For this review, take the finished solid that the model builds, in its own axes (mm). Face numbers are marked on the shaded views. A direction names the side the tool comes from. Give positions to 0.01 mm unless a question says otherwise; leave off trailing zeros. Order: outer loops, then holes, each group sorted by start corner. A loop starts at its lowest first (then second) coordinate and runs counter-clockwise, first axis right, second up.
Item 1: Consider section A-A (x = 0). Give the boundary of the cut face in (y, z).
Item 2: Machinability: for the marked faces 4, 5 and 6, which of the approach directions +Z, -Z, +X, -X, +Y, -Y give a long, thin tool a straight path to every point of the face, cutting with its end or side? Answer none if there is none.
Item 3: For P1, Ø2, axis at y = -0.5, z = -20.5, coming from the +X side; P2, Ø1, axis at x = 5, y = 1, coming from the +Z side; P3, Ø6, axis at y = -0.5, z = -13, coming from the +X side, all flat-tipped, find the tip position at first contact; note any pin that passes through.
Item 4: The part is to be moulded in two halves that separate along Z. For the marked faces 1, 2 and 3, say which applies: released by +Z, released by -Z, zero draft, split by the parting line, or undercut.
Item 5: Consider section B-B (z = -31). Give the boundary of the cut face in (x, y).
Item 6: Consider section D-D (x = -7). Give the boundary of the cut face in (y, z).
Item 7: For probe 1 along Z at (x, y) = (0, 0.25); probe 2 along X at (y, z) = (-4.5, -9.5); probe 3 along Z at (x, y) = (-4, -2.5), list the stretches that pass through material, from the lowest coordinate up.
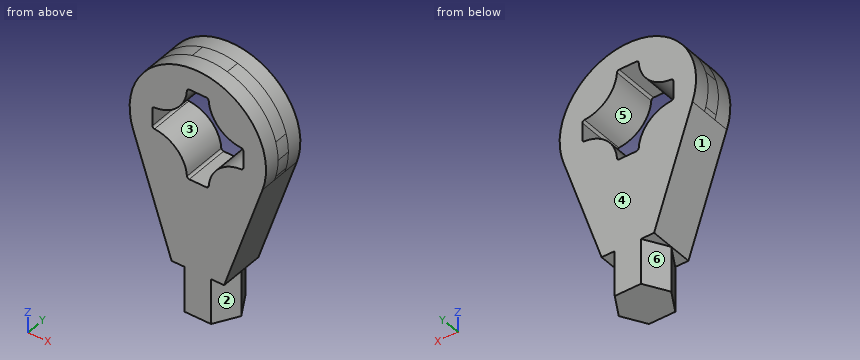
```python
from build123d import *

# Parameters (mm, degrees)
F1_DEPTH   = 3
F5_DEPTH   = 10
F7_DEPTH   = 3
F1_FACE1_R = 15
F8_DEPTH   = 3.5
F1_FACE_R  = 15
F9_DEPTH   = 3.5
F11_R      = 0.5


with BuildPart() as f1:
    # F0 (on Front) → F1 (new body)
    with BuildSketch(Plane.XZ):
        with BuildLine():
            Line((-10, -2.375), (-10, 2.375))
            ThreePointArc((-10, 2.375), (-12.3664158462, 2.7515035323), (-14.4991362367, 3.8438325133))
            ThreePointArc((-14.4991362367, 3.8438325133), (-15, 0), (-14.4991362367, -3.8438325133))
            ThreePointArc((-14.4991362367, -3.8438325133), (-12.3664158462, -2.7515035323), (-10, -2.375))
        make_face()
        with BuildLine():
            Line((-10, 10), (-2.375, 10))
            ThreePointArc((-2.375, 10), (-2.7515035323, 12.3664158462), (-3.8438325133, 14.4991362367))
            ThreePointArc((-3.8438325133, 14.4991362367), (-10.6066017178, 10.6066017178), (-14.4991362367, 3.8438325133))
            ThreePointArc((-14.4991362367, 3.8438325133), (-12.3664158462, 2.7515035323), (-10, 2.375))
            Line((-10, 2.375), (-10, 10))
        make_face()
        with BuildLine():
            ThreePointArc((-10, 2.375), (-4.6083107935, 4.6083107935), (-2.375, 10))
            Line((-2.375, 10), (-10, 10))
            Line((-10, 10), (-10, 2.375))
        make_face()
        with BuildLine():
            Line((-2.375, 10), (2.375, 10))
            ThreePointArc((2.375, 10), (2.7515035323, 12.3664158462), (3.8438325133, 14.4991362367))
            ThreePointArc((3.8438325133, 14.4991362367), (0, 15), (-3.8438325133, 14.4991362367))
            ThreePointArc((-3.8438325133, 14.4991362367), (-2.7515035323, 12.3664158462), (-2.375, 10))
        make_face()
        with BuildLine():
            Line((2.375, 10), (10, 10))
            Line((10, 10), (10, 2.375))
            ThreePointArc((10, 2.375), (12.3664158462, 2.7515035323), (14.4991362367, 3.8438325133))
            ThreePointArc((14.4991362367, 3.8438325133), (10.6066017178, 10.6066017178), (3.8438325133, 14.4991362367))
            ThreePointArc((3.8438325133, 14.4991362367), (2.7515035323, 12.3664158462), (2.375, 10))
        make_face()
        with BuildLine():
            ThreePointArc((14.4991362367, 3.8438325133), (12.3664158462, 2.7515035323), (10, 2.375))
            Line((10, 2.375), (10, -2.375))
            ThreePointArc((10, -2.375), (12.3664158462, -2.7515035323), (14.4991362367, -3.8438325133))
            ThreePointArc((14.4991362367, -3.8438325133), (14.8742570159, -1.9381636218), (15, 0))
            ThreePointArc((15, 0), (14.8742570159, 1.9381636218), (14.4991362367, 3.8438325133))
        make_face()
        with BuildLine():
            ThreePointArc((14.4991362367, -3.8438325133), (12.3664158462, -2.7515035323), (10, -2.375))
            Line((10, -2.375), (10, -10))
            Line((10, -10), (2.375, -10))
            ThreePointArc((2.375, -10), (2.7515035323, -12.3664158462), (3.8438325133, -14.4991362367))
            ThreePointArc((3.8438325133, -14.4991362367), (10.6066017178, -10.6066017178), (14.4991362367, -3.8438325133))
        make_face()
        with BuildLine():
            ThreePointArc((3.8438325133, -14.4991362367), (2.7515035323, -12.3664158462), (2.375, -10))
            Line((2.375, -10), (-2.375, -10))
            ThreePointArc((-2.375, -10), (-2.7515035323, -12.3664158462), (-3.8438325133, -14.4991362367))
            ThreePointArc((-3.8438325133, -14.4991362367), (0, -15), (3.8438325133, -14.4991362367))
        make_face()
        with BuildLine():
            Line((-10, -10), (-10, -2.375))
            ThreePointArc((-10, -2.375), (-12.3664158462, -2.7515035323), (-14.4991362367, -3.8438325133))
            ThreePointArc((-14.4991362367, -3.8438325133), (-10.6066017178, -10.6066017178), (-3.8438325133, -14.4991362367))
            ThreePointArc((-3.8438325133, -14.4991362367), (-2.7515035323, -12.3664158462), (-2.375, -10))
            Line((-2.375, -10), (-10, -10))
        make_face()
        with BuildLine():
            ThreePointArc((-2.375, -10), (-4.6083107935, -4.6083107935), (-10, -2.375))
            Line((-10, -2.375), (-10, -10))
            Line((-10, -10), (-2.375, -10))
        make_face()
        with BuildLine():
            Line((10, -10), (10, -2.375))
            ThreePointArc((10, -2.375), (4.6083107935, -4.6083107935), (2.375, -10))
            Line((2.375, -10), (10, -10))
        make_face()
        with BuildLine():
            Line((10, 2.375), (10, 10))
            Line((10, 10), (2.375, 10))
            ThreePointArc((2.375, 10), (4.6083107935, 4.6083107935), (10, 2.375))
        make_face()
    extrude(amount=F1_DEPTH)


with BuildPart() as f5:
    # F4 (on offset) → F5 (new body)
    with BuildSketch(Plane.XY.offset(-40)):
        Polygon((2.8867513459, 3.5), (-2.8867513459, 3.5), (-5.7735026919, -1.5), (-2.8867513459, -6.5), (2.8867513459, -6.5), (5.7735026919, -1.5), align=None)
    extrude(amount=F5_DEPTH)


with BuildPart() as f7:
    # F6 (on face) → F7 (new body, through all)
    with BuildSketch(Plane(origin=(0, 0, 0), x_dir=(-1, 0, 0), z_dir=(0, 1, 0))):
        with BuildLine():
            ThreePointArc((14.2238332207, -4.7626220204), (0, -15), (-14.2238332207, -4.7626220204))
            Line((-14.2238332207, -4.7626220204), (-5.7735026919, -30))
            Line((-5.7735026919, -30), (5.7735026919, -30))
            Line((5.7735026919, -30), (14.2238332207, -4.7626220204))
        make_face()
    extrude(amount=-F7_DEPTH)


with BuildPart() as f8:
    # F7_face (on face) + F1_face1 (on face) → F8 (new body, through all)
    with BuildSketch(Plane(origin=(0, 0, -20.4204827201), x_dir=(-1, 0, 0), z_dir=(0, 1, 0))):
        with BuildLine():
            ThreePointArc((14.2238332207, 15.6578606997), (0, 5.4204827201), (-14.2238332207, 15.6578606997))
            Line((-14.2238332207, 15.6578606997), (-5.7735026919, -9.5795172799))
            Line((-5.7735026919, -9.5795172799), (5.7735026919, -9.5795172799))
            Line((5.7735026919, -9.5795172799), (14.2238332207, 15.6578606997))
        make_face()
    with BuildSketch(Plane(origin=(0, 0, 0), x_dir=(1, 0, 0), z_dir=(0, 1, 0))):
        Circle(F1_FACE1_R)
        with BuildLine():
            ThreePointArc((-2.375, -10), (-4.6083107935, -4.6083107935), (-10, -2.375))
            Line((-10, -2.375), (-10, 2.375))
            ThreePointArc((-10, 2.375), (-4.6083107935, 4.6083107935), (-2.375, 10))
            Line((-2.375, 10), (2.375, 10))
            ThreePointArc((2.375, 10), (4.6083107935, 4.6083107935), (10, 2.375))
            Line((10, 2.375), (10, -2.375))
            ThreePointArc((10, -2.375), (4.6083107935, -4.6083107935), (2.375, -10))
            Line((2.375, -10), (-2.375, -10))
        make_face(mode=Mode.SUBTRACT)
    extrude(amount=F8_DEPTH)


with BuildPart() as f9:
    # F1_face (on face) + F7_face1 (on face) → F9 (new body, through all)
    with BuildSketch(Plane.XZ.offset(3)):
        Circle(F1_FACE_R)
        with BuildLine():
            ThreePointArc((-10, 2.375), (-4.6083107935, 4.6083107935), (-2.375, 10))
            Line((-2.375, 10), (2.375, 10))
            ThreePointArc((2.375, 10), (4.6083107935, 4.6083107935), (10, 2.375))
            Line((10, 2.375), (10, -2.375))
            ThreePointArc((10, -2.375), (4.6083107935, -4.6083107935), (2.375, -10))
            Line((2.375, -10), (-2.375, -10))
            ThreePointArc((-2.375, -10), (-4.6083107935, -4.6083107935), (-10, -2.375))
            Line((-10, -2.375), (-10, 2.375))
        make_face(mode=Mode.SUBTRACT)
    with BuildSketch(Plane(origin=(0, -3, -20.4204827201), x_dir=(-1, 0, 0), z_dir=(0, -1, 0))):
        with BuildLine():
            ThreePointArc((-14.2238332207, -15.6578606997), (0, -5.4204827201), (14.2238332207, -15.6578606997))
            Line((14.2238332207, -15.6578606997), (5.7735026919, 9.5795172799))
            Line((5.7735026919, 9.5795172799), (-5.7735026919, 9.5795172799))
            Line((-5.7735026919, 9.5795172799), (-14.2238332207, -15.6578606997))
        make_face()
    extrude(amount=F9_DEPTH)


with BuildPart() as f5_1:
    add(f5.part)

    # F10: union F8, F7, F9, F1
    add(f8.part)
    add(f7.part)
    add(f9.part)
    add(f1.part)

    # F11
    f11_edges = [f5_1.edges().sort_by_distance(p)[0] for p in [
        (10, -1.5, -2.375),
        (10, -1.5, 2.375),
        (2.375, -1.5, -10),
        (-2.375, -1.5, -10),
        (-10, -1.5, -2.375),
        (-10, -1.5, 2.375),
        (-2.375, -1.5, 10),
        (2.375, -1.5, 10),
    ]]
    fillet(f11_edges, radius=F11_R)


solid = f5_1.part
```
Resolved:
1. outline: (-6.5, -40) - (3.5, -40) - (3.5, -10) - (-6.5, -10) - close; (-6.5, 10) - (3.5, 10) - (3.5, 15) - (-6.5, 15) - close
2. face 4: +Z, -Z, +X, -X, +Y
2. face 5: +Y, -Y
2. face 6: -Z, -X, +Y
3. P1: stops at x = 9.29
3. P2: stops at z = 14.31
3. P3: stops at x = 12.47
4. face 1: released by -Z
4. face 2: zero draft
4. face 3: undercut
5. outline: (-5.77, -1.5) - (-2.89, -6.5) - (2.89, -6.5) - (5.77, -1.5) - (2.89, 3.5) - (-2.89, 3.5) - close
6. outline: (-6.5, -26.34) - (3.5, -26.34) - (3.5, -2.99) - (-6.5, -2.99) - close; (-6.5, 2.99) - (3.5, 2.99) - (3.5, 13.27) - (-6.5, 13.27) - close
7. probe 1: z = -40 to -10, 10 to 15
7. probe 2: x = -12.64 to -2.39, 2.39 to 12.64
7. probe 3: z = -40 to -5.29, 5.29 to 14.46
